```python
from build123d import *

# Parameters (mm, degrees)
F1_DEPTH  = 3.048
F2_W      = 115.7319251503
F2_H      = 3.048
F3_DEPTH  = 3.049
F5_W      = 2.54
F5_H      = 0.254
F6_DEPTH  = 3.049
F8_DEPTH  = 3.048
F9_W      = 3.175
F9_H      = 1.524
F10_DEPTH = 1.5875
F11_W     = 38.1
F11_H     = 3.048
F12_DEPTH = 3.048


with BuildPart() as f1:
    # F0 (on Top) → F1 (new body)
    with BuildSketch(Plane.XY):
        with BuildLine():
            Line((-79.9225977639, 113.03), (-137.8481502717, 12.7))
            ThreePointArc((-137.8481502717, 12.7), (-141.2511050156, 0), (-137.8481502717, -12.7))
            Line((-137.8481502717, -12.7), (-79.9225977639, -113.03))
            ThreePointArc((-79.9225977639, -113.03), (-70.6255525078, -122.3270452561), (-57.9255525078, -125.73))
            Line((-57.9255525078, -125.73), (57.9255525078, -125.73))
            ThreePointArc((57.9255525078, -125.73), (70.6255525078, -122.3270452561), (79.9225977639, -113.03))
            Line((79.9225977639, -113.03), (137.8481502717, -12.7))
            ThreePointArc((137.8481502717, -12.7), (141.2511050156, 0), (137.8481502717, 12.7))
            Line((137.8481502717, 12.7), (79.9225977639, 113.03))
            ThreePointArc((79.9225977639, 113.03), (70.6255525078, 122.3270452561), (57.9255525078, 125.73))
            Line((57.9255525078, 125.73), (-57.9255525078, 125.73))
            ThreePointArc((-57.9255525078, 125.73), (-70.6255525078, 122.3270452561), (-79.9225977639, 113.03))
        make_face()
    extrude(amount=F1_DEPTH)

    # F2 (on face) → F3 (cut, through all)
    with BuildSketch(Plane.XY.offset(3.048)):
        Polygon((-135.0389296821, -11.215712791), (-77.1729671069, -111.4425), (-74.5333216761, -109.9185), (-132.3992842513, -9.6917127909), align=None)
        Polygon((-77.2325570395, 111.339287209), (-135.0985196147, 11.1125), (-132.4588741839, 9.5885), (-74.5929116088, 109.8152872091), align=None)
        with Locations((-0.0595899326, 121.031)):
            Rectangle(F2_W, F2_H)
        Polygon((135.0389296821, 11.215712791), (77.1729671069, 111.4425), (74.5333216761, 109.9185), (132.3992842513, 9.691712791), align=None)
        Polygon((77.2325570395, -111.339287209), (135.0985196147, -11.1125), (132.4588741839, -9.5885), (74.5929116088, -109.815287209), align=None)
        with Locations((0.0595899326, -121.031)):
            Rectangle(F2_W, F2_H)
    extrude(amount=-F3_DEPTH, mode=Mode.SUBTRACT)

    # F5 (on face) → F6 (cut, through all)
    with BuildSketch(Plane.XY.offset(3.048)):
        with Locations((-9.525, -125.603)):
            Rectangle(F5_W, F5_H)
        with Locations((9.5845899326, -125.603)):
            Rectangle(F5_W, F5_H)
    extrude(amount=-F6_DEPTH, mode=Mode.SUBTRACT)

    # F7 (on face) → F8 (join)
    with BuildSketch(Plane.XY.offset(3.048)):
        with BuildLine():
            Line((-73.3234841871, 124.46), (-79.9225977639, 113.03))
            Line((-79.9225977639, 113.03), (-57.9255525078, 125.73))
            Line((-57.9255525078, 125.73), (-71.1237796615, 125.73))
            ThreePointArc((-71.1237796615, 125.73), (-72.3937796615, 125.3897045256), (-73.3234841871, 124.46))
        make_face()
        with BuildLine():
            ThreePointArc((-137.8481502717, -12.7), (-141.2511050156, 0), (-137.8481502717, 12.7))
            Line((-137.8481502717, 12.7), (-144.4472638486, 1.27))
            ThreePointArc((-144.4472638486, 1.27), (-144.7875593229, 0), (-144.4472638486, -1.27))
            Line((-144.4472638486, -1.27), (-137.8481502717, -12.7))
        make_face()
        with BuildLine():
            ThreePointArc((-57.9255525078, -125.73), (-70.6255525078, -122.3270452561), (-79.9225977639, -113.03))
            Line((-79.9225977639, -113.03), (-73.3234841871, -124.46))
            ThreePointArc((-73.3234841871, -124.46), (-72.3937796615, -125.3897045256), (-71.1237796615, -125.73))
            Line((-71.1237796615, -125.73), (-57.9255525078, -125.73))
        make_face()
        with BuildLine():
            Line((73.3234841871, -124.46), (79.9225977639, -113.03))
            ThreePointArc((79.9225977639, -113.03), (70.6255525078, -122.3270452561), (57.9255525078, -125.73))
            Line((57.9255525078, -125.73), (71.1237796615, -125.73))
            ThreePointArc((71.1237796615, -125.73), (72.3937796615, -125.3897045256), (73.3234841871, -124.46))
        make_face()
        with BuildLine():
            Line((144.4472638486, 1.27), (137.8481502717, 12.7))
            ThreePointArc((137.8481502717, 12.7), (141.2511050156, 0), (137.8481502717, -12.7))
            Line((137.8481502717, -12.7), (144.4472638486, -1.27))
            ThreePointArc((144.4472638486, -1.27), (144.7875593229, 0), (144.4472638486, 1.27))
        make_face()
        with BuildLine():
            Line((71.1237796615, 125.73), (57.9255525078, 125.73))
            ThreePointArc((57.9255525078, 125.73), (70.6255525078, 122.3270452561), (79.9225977639, 113.03))
            Line((79.9225977639, 113.03), (73.3234841871, 124.46))
            ThreePointArc((73.3234841871, 124.46), (72.3937796615, 125.3897045256), (71.1237796615, 125.73))
        make_face()
    extrude(amount=-F8_DEPTH)

    # F9 (on face) → F10 (cut)
    with BuildSketch(Plane.XY.offset(3.048)):
        with BuildLine():
            Line((-57.9255525078, 117.983), (-57.9255525078, 119.507))
            ThreePointArc((-57.9255525078, 119.507), (-67.5657049473, 116.9079552121), (-74.5929116088, 109.8152872091))
            Line((-74.5929116088, 109.8152872091), (-73.2684038811, 109.0614601206))
            ThreePointArc((-73.2684038811, 109.0614601206), (-66.7996293906, 115.5904939256), (-57.9255525078, 117.983))
        make_face()
        with Locations((-56.3380525078, 118.745)):
            Rectangle(F9_W, F9_H)
        Polygon((-73.2684038811, 109.0614601206), (-74.5929116088, 109.8152872091), (-76.1804116088, 107.065656552), (-74.8388469782, 106.3021217395), align=None)
        with BuildLine():
            Line((73.2182344036, 109.1483562046), (74.5333216761, 109.9185))
            ThreePointArc((74.5333216761, 109.9185), (67.446525082, 116.9398894425), (57.8063726425, 119.507))
            Line((57.8063726425, 119.507), (57.8063726425, 117.983))
            ThreePointArc((57.8063726425, 117.983), (66.6886079177, 115.6177179059), (73.2182344036, 109.1483562046))
        make_face()
        Polygon((76.1208216761, 107.168869343), (74.5333216761, 109.9185), (73.2182344036, 109.1483562046), (74.801024176, 106.406883901), align=None)
        with Locations((56.2188726425, 118.745)):
            Rectangle(F9_W, F9_H)
        with BuildLine():
            Line((-131.1390514686, 8.8265), (-132.4588741839, 9.5885))
            ThreePointArc((-132.4588741839, 9.5885), (-135.0281115918, -0.0596393029), (-132.3992842513, -9.6917127909))
            Line((-132.3992842513, -9.6917127909), (-131.0841969788, -8.9215689955))
            ThreePointArc((-131.0841969788, -8.9215689955), (-133.5041188708, -0.0549290528), (-131.1390514686, 8.8265))
        make_face()
        Polygon((-130.8713741839, 12.338130657), (-132.4588741839, 9.5885), (-131.1390514686, 8.8265), (-129.563948664, 11.5940256944), align=None)
        Polygon((-131.0841969788, -8.9215689955), (-132.3992842513, -9.6917127909), (-130.8117842513, -12.4413434479), (-129.4919867512, -11.679358006), align=None)
        with BuildLine():
            Line((-73.2134989608, -109.1565), (-74.5333216761, -109.9185))
            ThreePointArc((-74.5333216761, -109.9185), (-67.4624066445, -116.9675945149), (-57.8063726425, -119.507))
            Line((-57.8063726425, -119.507), (-57.8157930976, -117.983029116))
            ThreePointArc((-57.8157930976, -117.983029116), (-66.7044894803, -115.6454229784), (-73.2134989608, -109.1565))
        make_face()
        Polygon((-76.1208216761, -107.1688693429), (-74.5333216761, -109.9185), (-73.2134989608, -109.1565), (-74.8009989608, -106.4068693429), align=None)
        Polygon((-57.8157930976, -117.983029116), (-57.8063726425, -119.507), (-54.6313726425, -119.507), (-54.6313726425, -117.983029116), align=None)
        with BuildLine():
            Line((57.9161320527, -117.983029116), (57.9255525078, -119.507))
            ThreePointArc((57.9255525078, -119.507), (67.5496524319, -116.8803488392), (74.5929116088, -109.815287209))
            Line((74.5929116088, -109.815287209), (73.2730888934, -109.053287209))
            ThreePointArc((73.2730888934, -109.053287209), (66.7835768752, -115.5628875527), (57.9161320527, -117.983029116))
        make_face()
        Polygon((54.7505525078, -119.507), (57.9255525078, -119.507), (57.9161320527, -117.983029116), (54.7505525078, -117.983029116), align=None)
        Polygon((73.2730888934, -109.053287209), (74.5929116088, -109.815287209), (76.1804116088, -107.065656552), (74.8605888934, -106.303656552), align=None)
        with BuildLine():
            Line((131.1343664563, -8.8346729115), (132.4588741839, -9.5885))
            ThreePointArc((132.4588741839, -9.5885), (134.9961775139, 0.0595406033), (132.3992842513, 9.691712791))
            Line((132.3992842513, 9.691712791), (131.0794615359, 8.929712791))
            ThreePointArc((131.0794615359, 8.929712791), (133.4721847929, 0.0548303532), (131.1343664563, -8.8346729115))
        make_face()
        Polygon((130.8713741839, -12.338130657), (132.4588741839, -9.5885), (131.1343664563, -8.8346729115), (129.5515766838, -11.576145215), align=None)
        Polygon((131.0794615359, 8.929712791), (132.3992842513, 9.691712791), (130.8117842513, 12.441343448), (129.4919615359, 11.679343448), align=None)
    extrude(amount=-F10_DEPTH, mode=Mode.SUBTRACT)

    # F11 (on face) → F12 (join, through all)
    with BuildSketch(Plane.XY.offset(3.048)):
        with Locations((-0.0595899326, 121.031)):
            Rectangle(F11_W, F11_H)
        Polygon((-96.6405383271, 77.7236775466), (-115.6905383271, 44.7281096624), (-113.0508928964, 43.2041096624), (-94.0008928964, 76.1996775466), align=None)
        Polygon((-115.6309483945, -44.8313224534), (-96.5809483945, -77.8268903376), (-93.9413029637, -76.3028903376), (-112.9913029637, -43.3073224534), align=None)
        with Locations((0.0595899326, -121.031)):
            Rectangle(F11_W, F11_H)
        Polygon((96.6405383271, -77.7236775466), (115.6905383271, -44.7281096624), (113.0508928964, -43.2041096624), (94.0008928964, -76.1996775466), align=None)
        Polygon((115.6309483945, 44.8313224534), (96.5809483945, 77.8268903376), (93.9413029637, 76.3028903376), (112.9913029637, 43.3073224534), align=None)
    extrude(amount=-F12_DEPTH)


solid = f1.part
```
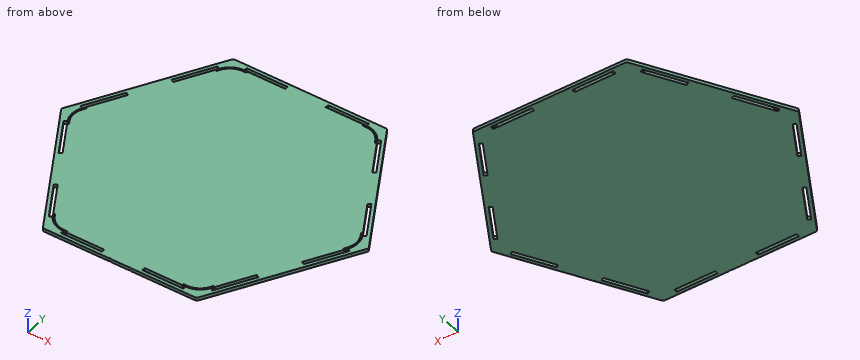
The model under review builds one solid part; all positions refer to its coordinate system, in mm. Give positions to 0.01 mm unless a question says otherwise; leave off trailing zeros. Loops run counter-clockwise (first coordinate to the right, second up) from the corner with the lowest first, then second, coordinate; pieces in that order, holes last. Notation, with made-up numbers: (17, 87) - (41, 87) arc R17 ccw to (41, 115) - close; hole circle Ø10 at (49.5, 12). An arc over 180 degrees is marked (long way). Answer as a JSON object with one key per item and string values.
Q1. Add section D-D on x = -101.5. State the section outline as (y, z) points, plus the area to 3 significant figures.
Worked out:
{"outline": "(-75.66, 0) - (75.66, 0) - (75.66, 3.05) - (-75.66, 3.05) - close", "area": "461 mm^2"}
Q2. To check wall thickness, follow line 1 along Y through (x, z) = (22, 0.7) (3 decimals); line 2 along X through (y, z) = (-85, 1); line 3 along Y through (x, z) = (84.5, 1.85). State the ranges of each line that lie inside material, in increasing order.
Worked out:
{"line 1": "y = -125.73 to -122.555, -119.507 to 119.507, 122.555 to 125.73", "line 2": "x = -96.11 to -92.44, -88.92 to 88.92, 92.44 to 96.11", "line 3": "y = -105.1 to -98.75, -92.66 to 92.66, 98.75 to 105.1"}
Q3. Add section A-A on x = 23.5. State the section outline as (y, z) points (3 decimals), plus the area to 3 significant figures.
Worked out:
{"outline": "(-125.73, 0) - (-122.555, 0) - (-122.555, 3.048) - (-125.73, 3.048) - close; (-119.507, 0) - (119.507, 0) - (119.507, 3.048) - (-119.507, 3.048) - close; (122.555, 0) - (125.73, 0) - (125.73, 3.048) - (122.555, 3.048) - close", "area": "748 mm^2"}
Q4. Add section C-C on z = 1. Count the separate pieces of the cut face and the enclosed holes in it, plus the area to 3 significant figures.
Worked out:
{"separate pieces": "1", "enclosed holes": "12", "area": "53,300 mm^2"}
Q5. Insertion check: pin 1 (1.5 mm diameter, centred on x = 109.5, z = 2.5, fed in from +Y); pin 2 (0.5 mm diameter, centred on y = -119, z = 2, fed in from -X); pin 3 (1.5 mm diameter, centred on y = -121, z = 1.5, fed in from -X); pin 4 (10 mm diameter, centred on x = 92.5, y = 82.5, fed in from +Z). Each pin has a flat end and moves straight along its axis. Give the tip position at first contact, or say it passes through.
Worked out:
{"pin 1": "stops at y = 63.1", "pin 2": "stops at x = -76.62", "pin 3": "stops at x = -75.75", "pin 4": "stops at z = 3.05"}
Q6. Add section B-B on y = -101. State the section outline as (x, z) points, plus the area to 3 significant figures.
Worked out:
{"outline": "(-86.87, 0) - (-83.2, 0) - (-83.2, 3.05) - (-86.87, 3.05) - close; (-79.68, 0) - (79.68, 0) - (79.68, 3.05) - (-79.68, 3.05) - close; (83.2, 0) - (86.87, 0) - (86.87, 3.05) - (83.2, 3.05) - close", "area": "508 mm^2"}
